Design review of the part built by this model. Coordinates are the model's own, in mm. Face numbers are marked on the shaded views. A direction names the side the tool comes from. Give positions to 0.01 mm unless a question says otherwise; leave off trailing zeros. Loops run counter-clockwise (first coordinate to the right, second up) from the corner with the lowest first, then second, coordinate; pieces in that order, holes last. Notation, with made-up numbers: (9, 59) -> (54, 59) arc R17 ccw to (54, 63) -> close; hole circle Ø3 at (5.5, -14.5). An arc over 180 degrees is marked (long way). Use a Markdown table: item, result. Add a question column.
1. For the marked faces 4 and 5, list the 3-axis set-ups (+Z, -Z, +X, -X, +Y, -Y) from which the entire face can be reached by the end or side of a thin tool; tool diameter is ignored.
2. Add section C-C (x = 3.5). State the section outline as (y, z) points.
3. Add section D-D (y = 14). State the section outline as (x, z) points, and give its area (3 significant figures).
4. To check wall thickness, follow line 1 (Y direction, x = 5.75, z = 7); line 2 (Y direction, x = 3.75, z = 15.75); line 3 (X direction, y = 17.5, z = 10). State the ranges of each line that lie inside material, in increasing order.
5. Draft analysis for pull direction Y (two halves, no side actions). For the marked faces 1, 2 and 3, state which applies: pulls with the +Y half, pulls with the -Y half, needs draft (parallel to the pull), parting line crosses it, or undercut.
6. Add section B-B (z = 10). State the section outline as (x, y) points, and give its area (3 significant figures).
7. Add section A-A (x = 5.25). State the section outline as (y, z) points.
8. For pin 1 Ø6 at (x, z) = (1, 7.5) entering from -Y; pin 2 Ø1.5 at (x, z) = (2, 11) entering from +Y; pin 3 Ø7.5 at (y, z) = (16.5, 5) entering from -X, all flat-tipped, find the tip position at first contact; note any pin that passes through.
```python
from build123d import *

# Parameters (mm, degrees)
BOSS_EXTRUDE1_DEPTH = 16
FILLET1_R           = 5


with BuildPart() as part:
    # Sketch1 → Boss-Extrude1 (new body)
    with BuildSketch(Plane.XY):
        Polygon((0, 0), (10, 0), (10, 23), (0, 23), (0, 19), (6, 19), (6, 12), (0, 12), align=None)
    extrude(amount=BOSS_EXTRUDE1_DEPTH)

    # Fillet1
    # the kernel refuses this fillet: 5 mm, written as the material it takes off along each edge
    with BuildSketch(Plane(origin=(0, 23, -12.247448714), x_dir=(1, 0, 0), z_dir=(0, 0, 1))) as fillet1_piece_1:
        with BuildLine():
            CenterArc((4.898979486, -5), FILLET1_R, 90, 78.463040967)
            Line((0, -4), (-0.09797959, -3.98))
            ThreePointArc((-0.09797959, -3.98), (-0.1, -2), (-0.1, 0))
            Line((-0.1, 0), (0, 0.1))
            Line((0, 0.1), (4.898979486, 0.1))
            Line((4.898979486, 0.1), (4.898979486, 0))
        make_face()
    extrude(amount=40.494897428, mode=Mode.SUBTRACT)


solid = part.part
```
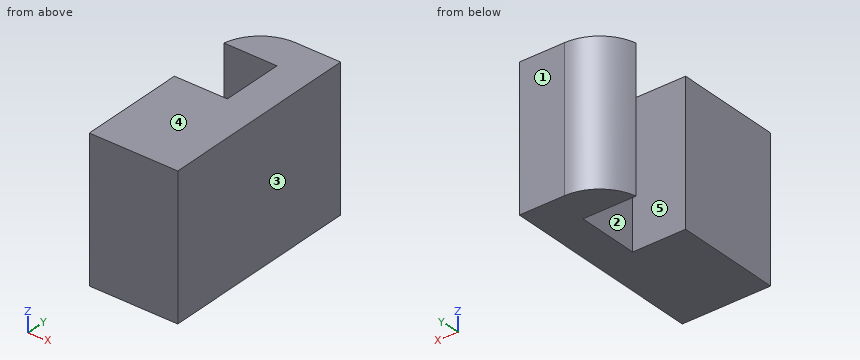
Taken from the geometry:
| question | item | result |
|---|---|---|
| 1 | face 4 | +Z, +X, -X, +Y, -Y |
| 1 | face 5 | +Z, -Z, -X |
| 2 | outline | (0, 0) -> (12, 0) -> (12, 16) -> (0, 16) -> close; (19, 0) -> (22.8, 0) -> (22.8, 16) -> (19, 16) -> close |
| 3 | outline | (6, 0) -> (10, 0) -> (10, 16) -> (6, 16) -> close |
| 3 | area | 64.0 mm^2 |
| 4 | line 1 | y = 0 to 12, 19 to 23 |
| 4 | line 2 | y = 0 to 12, 19 to 22.87 |
| 4 | line 3 | x = 6 to 10 |
| 5 | face 1 | pulls with the +Y half |
| 5 | face 2 | undercut |
| 5 | face 3 | needs draft |
| 6 | outline | (0, 0) -> (10, 0) -> (10, 23) -> (4.9, 23) arc R5 ccw to (0, 19) -> (6, 19) -> (6, 12) -> (0, 12) -> close |
| 6 | area | 183 mm^2 |
| 7 | outline | (0, 0) -> (12, 0) -> (12, 16) -> (0, 16) -> close; (19, 0) -> (23, 0) -> (23, 16) -> (19, 16) -> close |
| 8 | pin 1 | stops at y = 0 |
| 8 | pin 2 | stops at y = 22.51 |
| 8 | pin 3 | stops at x = 0 |
